For this review, use the dimensioned drawing (mm, ordinates from the lowest corner) and the shaded views. A direction names the side the tool comes from. Coordinates: 2 decimals unless noted, no trailing zeros. Order: outer loops, then holes, each group sorted by start corner. A loop starts at its lowest first (then second) coordinate and runs counter-clockwise, first axis right, second up. Notation, with made-up numbers: M 40,19.25 L 58,19.25 A33 cw 58,52.25 Z; hole C 81.25,-17 d7. An arc over 180 degrees is marked long. Answer in a Markdown table with one row per item.
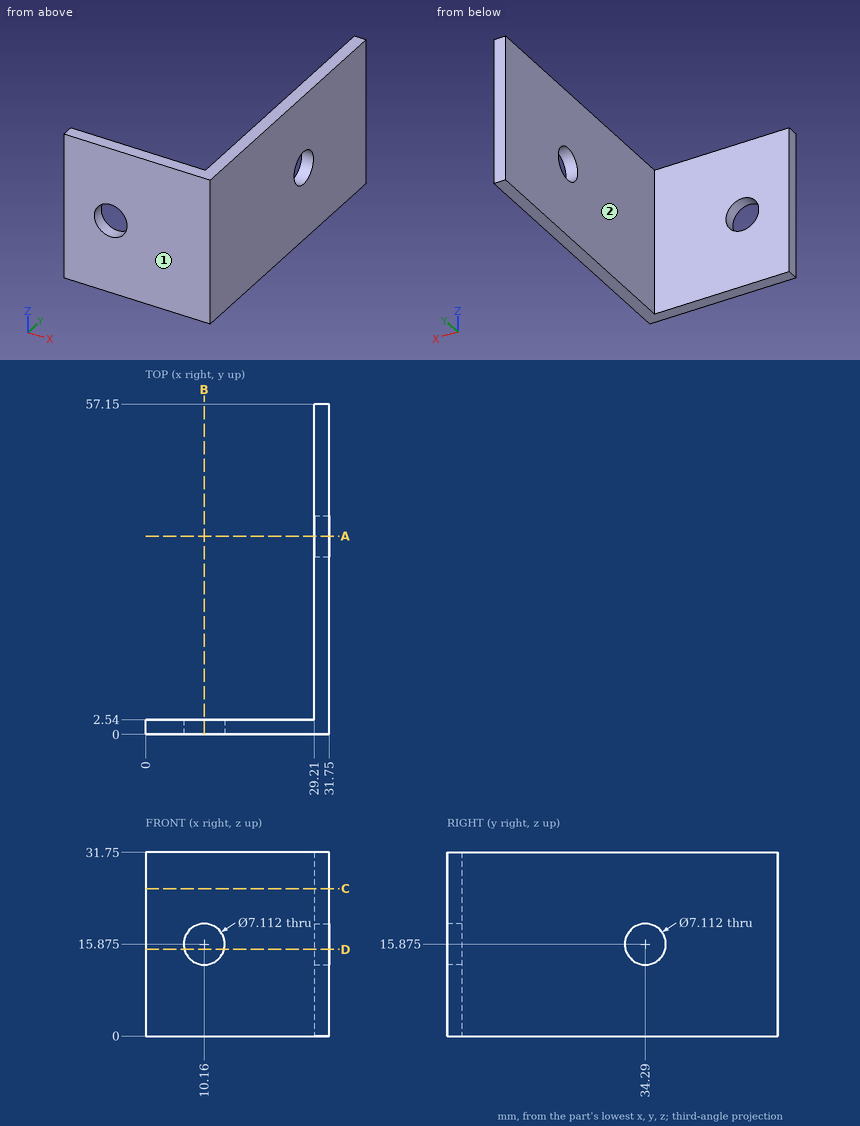
(1) For line 1 along Z through (x, y) = (10.16, 1.5); line 2 along X through (y, z) = (19.5, 16); line 3 along Y through (x, z) = (26, 2.5), list the stretches that pass through material, from the lowest coordinate up. Write a range as from..to.
Return value:
| item | result |
|---|---|
| line 1 | z = 0..12.32, 19.43..31.75 |
| line 2 | x = 29.21..31.75 |
| line 3 | y = 0..2.54 |
(2) For the marked faces 1 and 2, list the 3-axis set-ups (+Z, -Z, +X, -X, +Y, -Y) from which the entire face can be reached by the end or side of a thin tool; tool diameter is ignored.
Return value:
| item | result |
|---|---|
| face 1 | +Z, -Z, +X, -X, -Y |
| face 2 | +Z, -Z, -X, +Y |
(3) Add section D-D, the plane z = 15. Give the boundary of the cut face in (x, y), and give its area (3 significant figures).
Return value:
| item | result |
|---|---|
| outline | M 0,0 L 6.71,0 L 6.71,2.54 L 0,2.54 Z; M 13.61,0 L 31.75,0 L 31.75,30.84 L 29.21,30.84 L 29.21,2.54 L 13.61,2.54 Z; M 29.21,37.74 L 31.75,37.74 L 31.75,57.15 L 29.21,57.15 Z |
| area | 184 mm2 |
(4) Insertion check: pin 1 Ø6 at (x, y) = (24.5, 7.5) entering from -Z; pin 2 Ø3 at (y, z) = (8, 18) entering from -X; pin 3 Ø9 at (x, z) = (14.5, 17.5) entering from +Y. Each pin has a flat end and moves straight along its axis. Give the tip position at first contact, or say it passes through.
Return value:
| item | result |
|---|---|
| pin 1 | passes through |
| pin 2 | stops at x = 29.21 |
| pin 3 | stops at y = 2.54 |
(5) Add section A-A, the plane y = 34.29. Give the boundary of the cut face in (x, z), and give its area (3 significant figures).
Return value:
| item | result |
|---|---|
| outline | M 29.21,0 L 31.75,0 L 31.75,12.32 L 29.21,12.32 Z; M 29.21,19.43 L 31.75,19.43 L 31.75,31.75 L 29.21,31.75 Z |
| area | 62.6 mm2 |
(6) Add section B-B, the plane x = 10.16. Give the boundary of the cut face in (y, z), and give its area (3 significant figures).
Return value:
| item | result |
|---|---|
| outline | M 0,0 L 2.54,0 L 2.54,12.32 L 0,12.32 Z; M 0,19.43 L 2.54,19.43 L 2.54,31.75 L 0,31.75 Z |
| area | 62.6 mm2 |
(7) Add section C-C, the plane z = 25.5. Give the boundary of the cut face in (x, y).
Return value:
| item | result |
|---|---|
| outline | M 0,0 L 31.75,0 L 31.75,57.15 L 29.21,57.15 L 29.21,2.54 L 0,2.54 Z |
